Part model, mm, in its own coordinate system. Face numbers are marked on the shaded views. A direction names the side the tool comes from. Give positions to 0.01 mm unless a question says otherwise; leave off trailing zeros. Order: outer loops, then holes, each group sorted by start corner. A loop starts at its lowest first (then second) coordinate and runs counter-clockwise, first axis right, second up. Notation, with made-up numbers: M 21.5,-13.5 L 35.5,-13.5 A25 ccw 35.5,11.5 Z; hole C -39.75,22.25 d11. An arc over 180 degrees is marked long. Answer as a JSON object with one key per item and string values.
from build123d import *

# Parameters (mm, degrees)
ESQUISSE1_R                  = 74.5
BOSS_EXTRU_1_DEPTH           = 30
ESQUISSE3_R                  = 64
ENL_V_MAT_EXTRU_1_DEPTH      = 110.546793655
BOSS_EXTRU_2_DEPTH           = 30
ESQUISSE5_R                  = 1.6
ENL_V_MAT_EXTRU_2_DEPTH      = 120
R_P_TITION_CIRCULAIRE1_COUNT = 6
ENL_V_MAT_EXTRU_3_DEPTH      = 110.546793655
ENL_V_MAT_EXTRU_3_DEPTH_BACK = 110.546793655
ESQUISSE7_W                  = 12
ESQUISSE7_H                  = 16


with BuildPart() as part:
    # Esquisse1 → Boss.-Extru.1 (new body)
    with BuildSketch(Plane.XY):
        Circle(ESQUISSE1_R)
    extrude(amount=BOSS_EXTRU_1_DEPTH)

    # Esquisse3 → Enlèv. mat.-Extru.1 (cut, through all)
    with BuildSketch(Plane(origin=(0, 0, 0), x_dir=(-1, 0, 0), z_dir=(0, 0, -1))):
        Circle(ESQUISSE3_R)
    extrude(amount=-ENL_V_MAT_EXTRU_1_DEPTH, mode=Mode.SUBTRACT)

    # Esquisse4 → Boss.-Extru.2 (add)
    with BuildSketch(Plane(origin=(0, 0, 0), x_dir=(-1, 0, 0), z_dir=(0, 0, -1))):
        with BuildLine():
            ThreePointArc((-11.204980679, 63.011494253), (-8.166638415, 62.765293029), (-5.641396522, 61.05787037))
            ThreePointArc((-5.641396522, 61.05787037), (-3.097097656, 59.169334871), (0, 58.5))
            ThreePointArc((0, 58.5), (3.097097656, 59.169334871), (5.641396522, 61.05787037))
            ThreePointArc((5.641396522, 61.05787037), (8.166638415, 62.765293029), (11.204980679, 63.011494253))
            ThreePointArc((11.204980679, 63.011494253), (0, 64), (-11.204980679, 63.011494253))
        make_face()
    boss_extru_2 = extrude(amount=-BOSS_EXTRU_2_DEPTH)

    # Esquisse5 → Enlèv. mat.-Extru.2 (cut)
    with BuildSketch(Plane(origin=(0, 0, 0), x_dir=(-1, 0, 0), z_dir=(0, 0, -1))):
        with Locations((0, 66)):
            Circle(ESQUISSE5_R)
    enl_v_mat_extru_2 = extrude(amount=-ENL_V_MAT_EXTRU_2_DEPTH, mode=Mode.SUBTRACT)

    # Répétition circulaire1: Boss.-Extru.2, Enlèv. mat.-Extru.2 ×6 about axis
    r_p_tition_circulaire1_axis = Axis((0, 0, 0), (0, 0, 1))
    add([boss_extru_2.rotate(r_p_tition_circulaire1_axis, i * 360 / R_P_TITION_CIRCULAIRE1_COUNT) for i in range(1, R_P_TITION_CIRCULAIRE1_COUNT)])
    add([enl_v_mat_extru_2.rotate(r_p_tition_circulaire1_axis, i * 360 / R_P_TITION_CIRCULAIRE1_COUNT) for i in range(1, R_P_TITION_CIRCULAIRE1_COUNT)], mode=Mode.SUBTRACT)

    # Esquisse7 → Enlèv. mat.-Extru.3 (cut, two sides: drawn at the far end of the back side and taken through both)
    with BuildSketch(Plane(origin=(0, 0, 0), x_dir=(0, 0, -1), z_dir=(1, 0, 0)).offset(-ENL_V_MAT_EXTRU_3_DEPTH_BACK)):
        with Locations((-24, 0)):
            Rectangle(ESQUISSE7_W, ESQUISSE7_H)
    extrude(amount=ENL_V_MAT_EXTRU_3_DEPTH + ENL_V_MAT_EXTRU_3_DEPTH_BACK, mode=Mode.SUBTRACT)


solid = part.part
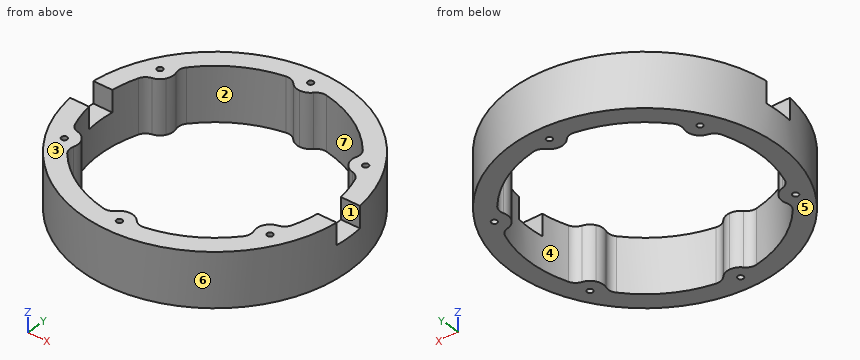
1. Probe line 1 along Y through (x, z) = (0, 7); line 2 along Y through (x, z) = (-0.5, 8.5); line 3 along X through (y, z) = (-50.5, 4.25). List the from-to ranges inside material, lowest first.
Worked answers:
{"line 1": "y = -74.5 to -67.6, -64.4 to -58.5, 58.5 to 64.4, 67.6 to 74.5", "line 2": "y = -74.5 to -67.52, -64.48 to -58.52, 58.52 to 64.48, 67.52 to 74.5", "line 3": "x = -54.77 to -39.32, 39.32 to 54.77"}
2. Cut at B-B on x = -34. Give the cut face in (y, z), plus the area to 3 significant figures.
Worked answers:
{"outline": "M -66.29,0 L -54.22,0 L -54.22,30 L -66.29,30 Z; M 54.22,0 L 66.29,0 L 66.29,30 L 54.22,30 Z", "area": "724 mm^2"}
3. Cut at C-C on z = 27.25. State how many separate pieces and enclosed holes the cut face has, plus the area to 3 significant figures.
Worked answers:
{"separate pieces": "2", "enclosed holes": "6", "area": "4,550 mm^2"}
4. Cut at A-A on y = 0. Give the cut face in (x, z).
Worked answers:
{"outline": "M -74.5,0 L -64,0 L -64,18 L -74.5,18 Z; M 64,0 L 74.5,0 L 74.5,18 L 64,18 Z"}
5. Pin check, flat tips, straight feed: P1, Ø11.5, axis at x = 66.5, z = 23, coming from the +Y side; P2, Ø5.5, axis at x = 70.5, y = -3.5, coming from the +Z side; P3, Ø2, axis at x = 29, z = 14.5, coming from the +Y side. Stop position of each tip, or through.
Worked answers:
{"P1": "stops at y = 43.12", "P2": "stops at z = 18", "P3": "stops at y = 69.04"}
6. Which spindle directions (+Z, -Z, +X, -X, +Y, -Y) get a long thin tool onto all of the face, cutting with end or side? Do the marked faces 1, 2 and 3. Say none if no direction does.
Worked answers:
{"face 1": "+Z, +X, -X", "face 2": "+Z, -Z", "face 3": "+Z, +X, -X, +Y, -Y"}
7. Two-plate mould, pull along X, no slides. Class the marked faces 4, 5, 6 and 7: +X half, -X half, draft (parallel to the pull), parting line (faces both ways), or undercut.
Worked answers:
{"face 4": "undercut", "face 5": "draft", "face 6": "parting line", "face 7": "undercut"}
